Geometry check sheet. Reference: the model listing, model coordinates, mm. A direction names the side the tool comes from. Give positions to 0.01 mm unless a question says otherwise; leave off trailing zeros. Loops run counter-clockwise (first coordinate to the right, second up) from the corner with the lowest first, then second, coordinate; pieces in that order, holes last. Notation, with made-up numbers: (74, 3.5) -> (90, 3.5) arc R19 cw to (90, 25.5) -> close; hole circle Ø8 at (52, 73). An arc over 180 degrees is marked (long way). Answer as a JSON object with one key per item and string values.
from build123d import *

# Parameters (mm, degrees)
BOSS_EXTRUDE1_DEPTH = 39
SKETCH2_R           = 4
CUT_EXTRUDE1_DEPTH  = 13.5
FILLET1_R           = 3


with BuildPart() as part:
    # Sketch1 → Boss-Extrude1 (new body)
    with BuildSketch(Plane.XY):
        Polygon((13.5, -12.5), (16.5, -7.5), (27.5, -7.5), (30.5, -12.5), (44, -12.5), (44, 0), (0, 0), (0, -12.5), align=None)
    extrude(amount=BOSS_EXTRUDE1_DEPTH)

    # Sketch2 → Cut-Extrude1 (cut, through all)
    with BuildSketch(Plane(origin=(0, 0, 0), x_dir=(1, 0, 0), z_dir=(0, 1, 0))):
        with Locations((7, -7)):
            Circle(SKETCH2_R)
        with Locations((37, -7)):
            Circle(SKETCH2_R)
        with Locations((37, -32)):
            Circle(SKETCH2_R)
        with Locations((7, -32)):
            Circle(SKETCH2_R)
    extrude(amount=-CUT_EXTRUDE1_DEPTH, mode=Mode.SUBTRACT)

    # Fillet1
    fillet1_edges = [part.edges().sort_by_distance(p)[0] for p in [
        (0, -6.25, 0),
        (44, -6.25, 39),
        (0, -6.25, 39),
        (44, -6.25, 0),
    ]]
    fillet(fillet1_edges, radius=FILLET1_R)


solid = part.part
1) Material ranges on line 1 along Z through (x, y) = (7, -7.5); line 2 along X through (y, z) = (-3, 32); line 3 along Z through (x, y) = (10.5, -6.5), recorded low to high. Write a range as from..to.
Geometry check:
{"line 1": "z = 0..3, 11..28, 36..39", "line 2": "x = 0..3, 11..33, 41..44", "line 3": "z = 0..5.06, 8.94..30.06, 33.94..39"}
2) Depth check by flat-ended pin: P1, Ø7, axis at x = 7, z = 32, coming from the -Y side; P2, Ø9, axis at x = 19.5, z = 18.5, coming from the -Y side; P3, Ø10.5, axis at x = 37, z = 32, coming from the -Y side. Enter the tip coordinate at first touch or a pass-through.
Geometry check:
{"P1": "passes through", "P2": "stops at y = -10", "P3": "stops at y = -12.5"}
3) Draft check along X on faces 1 (the face through (0, -6, 19)), 2 (the face through (29, -10, 19)), 3 (the face through (22, -6, 0)). Enter one of: pulls with the +X half, pulls with the -X half, needs draft (parallel to the pull), parting line crosses it, or undercut.
Geometry check:
{"face 1": "pulls with the -X half", "face 2": "undercut", "face 3": "needs draft"}
4) Section check B-B on z = 32. Record the cut outline in (x, y), plus the area to 3 significant figures.
Geometry check:
{"outline": "(0, -12.5) -> (3, -12.5) -> (3, 0) -> (0, 0) -> close; (11, -12.5) -> (13.5, -12.5) -> (16.5, -7.5) -> (27.5, -7.5) -> (30.5, -12.5) -> (33, -12.5) -> (33, 0) -> (11, 0) -> close; (41, -12.5) -> (44, -12.5) -> (44, 0) -> (41, 0) -> close", "area": "280 mm2"}
5) Section check A-A on y = -10.75. Record the cut outline in (x, z), plus the area to 3 significant figures.
Geometry check:
{"outline": "(0, 3) arc R3 ccw to (3, 0) -> (14.55, 0) -> (14.55, 39) -> (3, 39) arc R3 ccw to (0, 36) -> close; (29.45, 0) -> (41, 0) arc R3 ccw to (44, 3) -> (44, 36) arc R3 ccw to (41, 39) -> (29.45, 39) -> close; hole circle Ø8 at (7, 7); hole circle Ø8 at (7, 32); hole circle Ø8 at (37, 7); hole circle Ø8 at (37, 32)", "area": "926 mm2"}
6) Tool access check on faces 4 (the face through (22, 0, 19)), 5 (the face through (15, -10, 19)). Record the directions out of +Z, -Z, +X, -X, +Y, -Y that give a thin tool (end or side, any length) a straight path to the whole face; none if there is none.
Geometry check:
{"face 4": "+Z, -Z, +X, -X, +Y", "face 5": "+Z, -Z, -Y"}
7) Section check C-C on x = 37. Record the cut outline in (y, z), plus the area to 4 significant figures.
Geometry check:
{"outline": "(-12.5, 0) -> (0, 0) -> (0, 3) -> (-12.5, 3) -> close; (-12.5, 11) -> (0, 11) -> (0, 28) -> (-12.5, 28) -> close; (-12.5, 36) -> (0, 36) -> (0, 39) -> (-12.5, 39) -> close", "area": "287.5 mm2"}
8) Section check D-D on z = 11.5. Record the cut outline in (x, y).
Geometry check:
{"outline": "(0, -12.5) -> (13.5, -12.5) -> (16.5, -7.5) -> (27.5, -7.5) -> (30.5, -12.5) -> (44, -12.5) -> (44, 0) -> (0, 0) -> close"}
